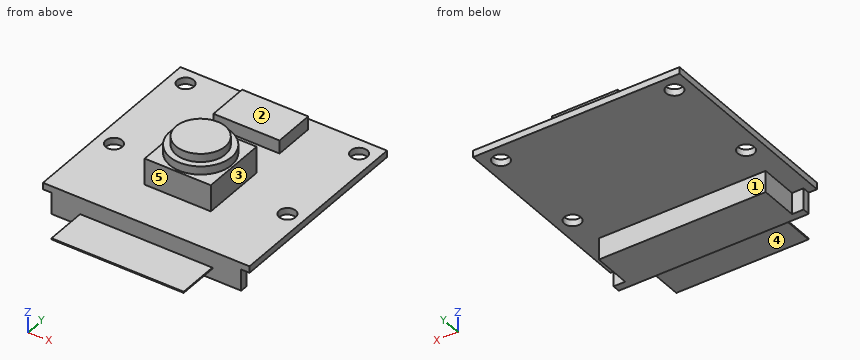
```python
from build123d import *

# Parameters (mm, degrees)
F0_W      = 25
F0_H      = 24
F1_DEPTH  = 0.8
F2_W      = 8
F2_H      = 8
F3_DEPTH  = 3.2
F4_R      = 3.75
F5_DEPTH  = 1
F6_R      = 3
F7_DEPTH  = 1
F9_D      = 2
F10_W     = 8
F10_H     = 5
F11_DEPTH = 1.6
F13_DEPTH = 2.6
F14_W     = 16
F14_H     = 0.15
F15_DEPTH = 5


with BuildPart() as f1:
    # F0 (on Top) → F1 (new body)
    with BuildSketch(Plane.XY):
        with Locations((0, 2.5)):
            Rectangle(F0_W, F0_H)
    extrude(amount=-F1_DEPTH)

    # F2 (on face) → F3 (join)
    with BuildSketch(Plane.XY):
        Rectangle(F2_W, F2_H)
    extrude(amount=F3_DEPTH)

    # F4 (on face) → F5 (join)
    with BuildSketch(Plane.XY.offset(3.2)):
        Circle(F4_R)
    extrude(amount=F5_DEPTH)

    # F6 (on face) → F7 (join)
    with BuildSketch(Plane.XY.offset(4.2)):
        Circle(F6_R)
    extrude(amount=F7_DEPTH)

    # F9 (through all)
    with Locations(Plane.XY):
        with Locations((-10.5, 12.5), (10.5, 12.5), (10.5, 0), (-10.5, 0)):
            Hole(F9_D / 2)

    # F10 (on face) → F11 (join)
    with BuildSketch(Plane.XY):
        with Locations((0, 10.5)):
            Rectangle(F10_W, F10_H)
    extrude(amount=F11_DEPTH)

    # F12 (on face) → F13 (join)
    with BuildSketch(Plane(origin=(0, 0, -0.8), x_dir=(1, 0, 0), z_dir=(0, 0, -1))):
        Polygon((11.5, 9.5), (-11.5, 9.5), (-11.5, 8.6), (-10.1, 8.6), (-10.1, 4), (10.1, 4), (10.1, 8.6), (11.5, 8.6), align=None)
    extrude(amount=F13_DEPTH)

    # F14 (on face) → F15 (join)
    with BuildSketch(Plane.XZ.offset(9.5)):
        with Locations((0, -2.075)):
            Rectangle(F14_W, F14_H)
    extrude(amount=F15_DEPTH)


solid = f1.part
```
Work out the finished part from the listing and answer in its coordinate system (mm). Face numbers are marked on the shaded views. A direction names the side the tool comes from. Coordinates: 2 decimals unless noted, no trailing zeros. Loops run counter-clockwise (first coordinate to the right, second up) from the corner with the lowest first, then second, coordinate; pieces in that order, holes last. Notation, with made-up numbers: (-35.75, 5.5) - (10.25, 5.5) arc R29 cw to (10.25, 34.5) - close; hole circle Ø7 at (-4, 26). An arc over 180 degrees is marked (long way). Use a Markdown table: item, result.
Item 1: Given pin 1 Ø1 at (x, y) = (8, 0.5) entering from -Z; pin 2 Ø1.3 at (y, z) = (-5.5, -2.5) entering from -X; pin 3 Ø1.5 at (x, y) = (-4, -11.5) entering from -Z; pin 4 Ø3.5 at (x, z) = (-5.5, -2.5) entering from -Y, each flat-ended and moving along its own axis, determine where each tip first touches the part or whether it passes through.
Evaluation:
| item | result |
|---|---|
| pin 1 | stops at z = -0.8 |
| pin 2 | stops at x = -10.1 |
| pin 3 | stops at z = -2.15 |
| pin 4 | stops at y = -14.5 |
Item 2: Find section A-A, the plane z = 0.5. Determine the outline of the cut face in (x, y).
Evaluation:
| item | result |
|---|---|
| outline | (-4, -4) - (4, -4) - (4, 4) - (-4, 4) - close; (-4, 8) - (4, 8) - (4, 13) - (-4, 13) - close |
Item 3: Find section D-D, the plane x = 0. Determine the outline of the cut face in (y, z).
Evaluation:
| item | result |
|---|---|
| outline | (-14.5, -2.15) - (-9.5, -2.15) - (-9.5, -3.4) - (-4, -3.4) - (-4, -0.8) - (14.5, -0.8) - (14.5, 0) - (13, 0) - (13, 1.6) - (8, 1.6) - (8, 0) - (4, 0) - (4, 3.2) - (3.75, 3.2) - (3.75, 4.2) - (3, 4.2) - (3, 5.2) - (-3, 5.2) - (-3, 4.2) - (-3.75, 4.2) - (-3.75, 3.2) - (-4, 3.2) - (-4, 0) - (-9.5, 0) - (-9.5, -2) - (-14.5, -2) - close |
Item 4: For the marked faces 1, 2, 3, 4 and 5, determine the directions among +Z, -Z, +X, -X, +Y, -Y from which every point of the face is accessible in a straight line to the end or side of a thin tool.
Evaluation:
| item | result |
|---|---|
| face 1 | -Z, +X, -X, +Y |
| face 2 | +Z, +X, -X, +Y |
| face 3 | +Z, +X, +Y, -Y |
| face 4 | -Z, +X, -X, -Y |
| face 5 | +Z, +X, -X, -Y |
Item 5: Find section C-C, the plane x = 10.5. Determine the outline of the cut face in (y, z), and give its area (3 significant figures).
Evaluation:
| item | result |
|---|---|
| outline | (-9.5, -3.4) - (-8.6, -3.4) - (-8.6, -0.8) - (-1, -0.8) - (-1, 0) - (-9.5, 0) - close; (1, -0.8) - (11.5, -0.8) - (11.5, 0) - (1, 0) - close; (13.5, -0.8) - (14.5, -0.8) - (14.5, 0) - (13.5, 0) - close |
| area | 18.3 mm2 |
Item 6: Consider probe 1 along Y at (x, z) = (-10.5, -0.15); probe 2 along Z at (x, y) = (-7.75, -6); probe 3 along X at (y, z) = (-0.5, 1). Determine where each line is inside the solid, lowest interval first. Write a range as from..to.
Evaluation:
| item | result |
|---|---|
| probe 1 | y = -9.5..-1, 1..11.5, 13.5..14.5 |
| probe 2 | z = -3.4..0 |
| probe 3 | x = -4..4 |
Item 7: Find section B-B, the plane y = 0. Determine the outline of the cut face in (x, z), and give its area (3 significant figures).
Evaluation:
| item | result |
|---|---|
| outline | (-12.5, -0.8) - (-11.5, -0.8) - (-11.5, 0) - (-12.5, 0) - close; (-9.5, -0.8) - (9.5, -0.8) - (9.5, 0) - (4, 0) - (4, 3.2) - (3.75, 3.2) - (3.75, 4.2) - (3, 4.2) - (3, 5.2) - (-3, 5.2) - (-3, 4.2) - (-3.75, 4.2) - (-3.75, 3.2) - (-4, 3.2) - (-4, 0) - (-9.5, 0) - close; (11.5, -0.8) - (12.5, -0.8) - (12.5, 0) - (11.5, 0) - close |
| area | 55.9 mm2 |
